Read the model definition and answer for the solid it produces. Units are mm, in the model's axes. Face numbers are marked on the shaded views. Give positions to 0.01 mm unless a question says otherwise; leave off trailing zeros. Order: outer loops, then holes, each group sorted by start corner. A loop starts at its lowest first (then second) coordinate and runs counter-clockwise, first axis right, second up. Notation, with made-up numbers: (-34, 80.25) -> (5, 80.25) arc R10 cw to (5, 98.25) -> close; hole circle Ø11 at (11, 83). An arc over 180 degrees is marked (long way). One line per question, with ' | ' between items. Start each with the question number.
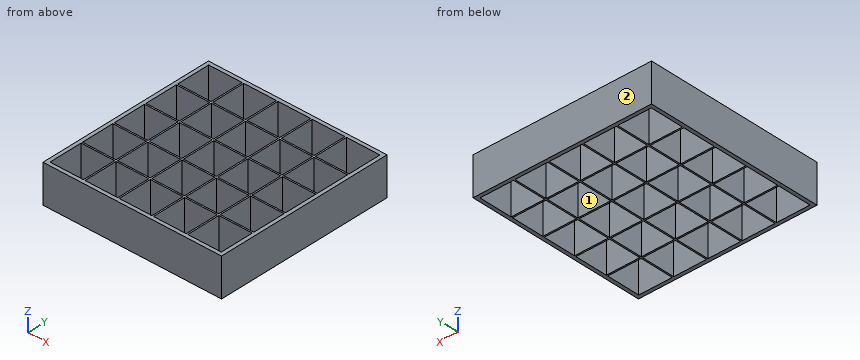
```python
from build123d import *

# Parameters (mm, degrees)
F0_W     = 1820
F0_H     = 1820
F0_W_2   = 341.7
F0_H_2   = 341.7
F0_W_3   = 334.2
F0_H_3   = 15
F0_W_4   = 15
F0_H_4   = 334.2
F1_DEPTH = 390


with BuildPart() as f1:
    # F0 (on Top) → F1 (new body)
    with BuildSketch(Plane.XY):
        Rectangle(F0_W, F0_H)
        with Locations((-702.15, -702.15)):
            Rectangle(F0_W_2, F0_H_2, mode=Mode.SUBTRACT)
        with Locations((702.15, -702.15)):
            Rectangle(F0_W_2, F0_H_2, mode=Mode.SUBTRACT)
        with Locations((-702.15, 702.15)):
            Rectangle(F0_W_2, F0_H_2, mode=Mode.SUBTRACT)
        Polygon((-531.3, 516.3), (-531.3, 531.3), (-516.3, 531.3), (-516.3, 873), (-182.1, 873), (-182.1, 531.3), (-167.1, 531.3), (-167.1, 873), (167.1, 873), (167.1, 531.3), (182.1, 531.3), (182.1, 873), (516.3, 873), (516.3, 531.3), (531.3, 531.3), (531.3, 516.3), (873, 516.3), (873, 182.1), (531.3, 182.1), (531.3, 167.1), (873, 167.1), (873, -167.1), (531.3, -167.1), (531.3, -182.1), (873, -182.1), (873, -516.3), (531.3, -516.3), (531.3, -531.3), (516.3, -531.3), (516.3, -873), (182.1, -873), (182.1, -531.3), (167.1, -531.3), (167.1, -873), (-167.1, -873), (-167.1, -531.3), (-182.1, -531.3), (-182.1, -873), (-516.3, -873), (-516.3, -531.3), (-531.3, -531.3), (-531.3, -516.3), (-873, -516.3), (-873, -182.1), (-531.3, -182.1), (-531.3, -167.1), (-873, -167.1), (-873, 167.1), (-531.3, 167.1), (-531.3, 182.1), (-873, 182.1), (-873, 516.3), align=None, mode=Mode.SUBTRACT)
        with Locations((702.15, 702.15)):
            Rectangle(F0_W_2, F0_H_2, mode=Mode.SUBTRACT)
        with Locations((-349.2, -523.8)):
            Rectangle(F0_W_3, F0_H_3)
        with Locations((-174.6, -523.8)):
            Rectangle(F0_W_4, F0_H_3)
        with Locations((0, -523.8)):
            Rectangle(F0_W_3, F0_H_3)
        with Locations((-174.6, -349.2)):
            Rectangle(F0_W_4, F0_H_4)
        with Locations((349.2, -523.8)):
            Rectangle(F0_W_3, F0_H_3)
        with Locations((174.6, -523.8)):
            Rectangle(F0_W_4, F0_H_3)
        with Locations((174.6, -349.2)):
            Rectangle(F0_W_4, F0_H_4)
        with Locations((523.8, -523.8)):
            Rectangle(F0_W_4, F0_H_3)
        with Locations((523.8, -349.2)):
            Rectangle(F0_W_4, F0_H_4)
        with Locations((523.8, 0)):
            Rectangle(F0_W_4, F0_H_4)
        with Locations((349.2, -174.6)):
            Rectangle(F0_W_3, F0_H_3)
        with Locations((523.8, -174.6)):
            Rectangle(F0_W_4, F0_H_3)
        with Locations((523.8, 349.2)):
            Rectangle(F0_W_4, F0_H_4)
        with Locations((523.8, 174.6)):
            Rectangle(F0_W_4, F0_H_3)
        with Locations((349.2, 174.6)):
            Rectangle(F0_W_3, F0_H_3)
        with Locations((349.2, 523.8)):
            Rectangle(F0_W_3, F0_H_3)
        with Locations((523.8, 523.8)):
            Rectangle(F0_W_4, F0_H_3)
        with Locations((-349.2, 523.8)):
            Rectangle(F0_W_3, F0_H_3)
        with Locations((-523.8, 523.8)):
            Rectangle(F0_W_4, F0_H_3)
        with Locations((-523.8, 349.2)):
            Rectangle(F0_W_4, F0_H_4)
        with Locations((-174.6, 349.2)):
            Rectangle(F0_W_4, F0_H_4)
        with Locations((-174.6, 523.8)):
            Rectangle(F0_W_4, F0_H_3)
        with Locations((0, 523.8)):
            Rectangle(F0_W_3, F0_H_3)
        with Locations((-523.8, 174.6)):
            Rectangle(F0_W_4, F0_H_3)
        with Locations((-349.2, 174.6)):
            Rectangle(F0_W_3, F0_H_3)
        with Locations((-523.8, 0)):
            Rectangle(F0_W_4, F0_H_4)
        with Locations((-174.6, 0)):
            Rectangle(F0_W_4, F0_H_4)
        with Locations((0, 174.6)):
            Rectangle(F0_W_3, F0_H_3)
        with Locations((-174.6, 174.6)):
            Rectangle(F0_W_4, F0_H_3)
        with Locations((-349.2, -174.6)):
            Rectangle(F0_W_3, F0_H_3)
        with Locations((-523.8, -349.2)):
            Rectangle(F0_W_4, F0_H_4)
        with Locations((-523.8, -174.6)):
            Rectangle(F0_W_4, F0_H_3)
        with Locations((0, -174.6)):
            Rectangle(F0_W_3, F0_H_3)
        with Locations((-174.6, -174.6)):
            Rectangle(F0_W_4, F0_H_3)
        with Locations((-523.8, -523.8)):
            Rectangle(F0_W_4, F0_H_3)
        with Locations((174.6, 0)):
            Rectangle(F0_W_4, F0_H_4)
        with Locations((174.6, -174.6)):
            Rectangle(F0_W_4, F0_H_3)
        with Locations((174.6, 349.2)):
            Rectangle(F0_W_4, F0_H_4)
        with Locations((174.6, 174.6)):
            Rectangle(F0_W_4, F0_H_3)
        with Locations((174.6, 523.8)):
            Rectangle(F0_W_4, F0_H_3)
    extrude(amount=F1_DEPTH)


solid = f1.part
```
Q1. Determine the mould class of the marked faces 1 and 2 for opening direction X: pulls with the +X half, pulls with the -X half, needs draft (parallel to the pull), parting line crosses it, or undercut.
Q2. A cutting plane is placed at A-A, the plane x = 583.5. Determine the outline of the cut face in (y, z).
Q3. A cutting plane is placed at C-C, the plane z = 74. Give the number of separate pieces and of enclosed holes in the cut face, then the cut area to 3 significant figures.
Q4. Find the intervals of material crossed by line 1 (X direction, y = 439.5, z = 132), in increasing order.
Geometry results:
1) face 1: undercut | face 2: needs draft
2) outline: (-910, 0) -> (-873, 0) -> (-873, 390) -> (-910, 390) -> close; (-531.3, 0) -> (-516.3, 0) -> (-516.3, 390) -> (-531.3, 390) -> close; (-182.1, 0) -> (-167.1, 0) -> (-167.1, 390) -> (-182.1, 390) -> close; (167.1, 0) -> (182.1, 0) -> (182.1, 390) -> (167.1, 390) -> close; (516.3, 0) -> (531.3, 0) -> (531.3, 390) -> (516.3, 390) -> close; (873, 0) -> (910, 0) -> (910, 390) -> (873, 390) -> close
3) separate pieces: 1 | enclosed holes: 25 | area: 470,000 mm²
4) line 1: -910 to -873, -531.3 to -516.3, -182.1 to -167.1, 167.1 to 182.1, 516.3 to 531.3, 873 to 910
